Autodesk Inventor part; units mm, degrees
ref_plane "YZ Plane" through (0, 0, 0) normal (1, 0, 0) x (0, 1, 0)
ref_plane "XZ Plane" through (0, 0, 0) normal (0, 1, 0) x (-1, 0, 0)
ref_plane "XY Plane" through (0, 0, 0) normal (0, 0, 1) x (1, 0, 0)
sketch "Sketch1" plane through (0, 0, 0) normal (0, 1, 0) x (-1, 0, 0)
  line L0 (17.0278, 0) -> (-10.5342, 0)
  line L1 (-10.5342, 0) -> (-10.5342, -20.5)
  line L2 (-10.5342, -20.5) -> (17.0278, -20.5)
  line L3 (17.0278, -20.5) -> (17.0278, 0)
  line L4 (4.9658, -15.846) -> (-7.0342, -15.846)
  line L5 (-7.0342, -15.846) -> (-7.0342, -10.846)
  line L6 (-7.0342, -10.846) -> (4.9658, -10.846)
  line L7 (4.9658, -10.846) -> (4.9658, -15.846)
  circle A0 centre (-6.0342, -14.846) radius 1
  circle A1 centre (3.9658, -14.846) radius 1
  circle A2 centre (3.9658, -11.846) radius 1
  circle A3 centre (-6.0342, -11.846) radius 1
  circle A4 centre (-8.5342, -18.5) radius 2
  line L8 (17.0278, -20.5) -> (-8.5342, -20.5)
  line L9 (-8.5342, -20.5) -> (-8.5342, -6.2)
  line L10 (-8.5342, -6.2) -> (17.0278, -6.2)
  line L11 (17.0278, -6.2) -> (17.0278, -20.5)
  line L12 (-10.5342, -20.5) -> (7.4658, -20.5)
  line L13 (7.4658, -20.5) -> (7.4658, -17.5)
  line L14 (7.4658, -17.5) -> (-10.5342, -17.5)
  line L15 (-10.5342, -17.5) -> (-10.5342, -20.5)
  line L16 (7.4658, -17.5) -> (17.0278, -17.5)
  line L17 (17.0278, -17.5) -> (17.0278, -8)
  line L18 (17.0278, -8) -> (7.4658, -8)
  line L19 (7.4658, -8) -> (7.4658, -17.5)
  circle A5 centre (17.0278, -12.75) radius 6.5
  line L20 (17.0278, -17.5) -> (21.4649, -17.5)
  line L21 (21.4649, -17.5) -> (21.4649, -8)
  line L22 (21.4649, -8) -> (17.0278, -8)
  line L23 (17.0278, -8) -> (17.0278, -17.5)
  circle A6 centre (5.6658, -8) radius 1.8
  line L24 (18.4658, -17.5) -> (13.4658, -17.5)
  line L25 (13.4658, -17.5) -> (13.4658, -13.6692)
  line L26 (13.4658, -13.6692) -> (18.4658, -13.6692)
  line L27 (18.4658, -13.6692) -> (18.4658, -17.5)
  circle A7 centre (19.4658, -16.5) radius 1
  circle A8 centre (17.4658, -14.6692) radius 1
  circle A9 centre (14.4658, -14.6692) radius 1
  circle A10 centre (12.4658, -16.5) radius 1
  line L28 (-8.5342, -17.5) -> (-10.5342, -17.5)
  line L29 (-10.5342, -17.5) -> (-10.5342, -6.2)
  line L30 (-10.5342, -6.2) -> (-8.5342, -6.2)
  line L31 (-8.5342, -6.2) -> (-8.5342, -17.5)
  point P0 (0, 0)
  point P1 (4.9658, -11.846)
  point P2 (4.9658, -14.846)
  point P3 (3.9658, -15.846)
  point P4 (-6.0342, -15.846)
  point P5 (-7.0342, -14.846)
  point P6 (-7.0342, -11.846)
  point P7 (-6.0342, -10.846)
  point P8 (3.9658, -10.846)
  point P9 (-8.5342, -16.5)
  point P10 (-8.5342, -20.5)
  point P11 (12.4658, -17.5)
  point P12 (13.4658, -16.5)
  point P13 (13.4658, -14.6692)
  point P14 (14.4658, -13.6692)
  point P15 (17.4658, -13.6692)
  point P16 (18.4658, -14.6692)
  point P17 (18.4658, -16.5)
  point P18 (19.4658, -17.5)
  point P19 (5.6658, -6.2)
  point P20 (-10.5342, -18.5)
  dimension "d26" = 13
  dimension "d1" = 20.5
  dimension "d2" = 0
  dimension "d3" = 12
  dimension "d4" = 5
  dimension "d5" = 4.654
  dimension "d6" = 3.5
  dimension "d7" = 2
  dimension "d8" = 2
  dimension "d9" = 2
  dimension "d10" = 2
  dimension "d11" = 1
  dimension "d12" = 1
  dimension "d13" = 1
  dimension "d14" = 1
  dimension "d15" = 1
  dimension "d16" = 1
  dimension "d17" = 1
  dimension "d18" = 1
  dimension "d19" = 4
  dimension "d20" = 2
  dimension "d21" = 14.3
  dimension "d22" = 18
  dimension "d23" = 3
  dimension "d24" = 9.5
  dimension "d25" = 9.562
  dimension "d27" = 1.8
  dimension "d28" = 5
  dimension "d29" = 8.5
  dimension "d30" = 2
  dimension "d31" = 2
  dimension "d32" = 2
  dimension "d33" = 2
  dimension "d34" = 1
  dimension "d35" = 1
  dimension "d36" = 1
  dimension "d37" = 1
  dimension "d38" = 1
  dimension "d39" = 1
  dimension "d40" = 1
  dimension "d41" = 1
extrude "Extrusion1" add sketch "Sketch1" along normal blind 3 contours L30 L9 A4 L14 L1 | A6 L19 L14 A4 L9 L10 | A6 | L14 A4 L1 | L22 L21 L20 A7 L27 L26 L3 | L3 L26 L25 A10 A5 L18 | A5 L21 | A5 A10 L16 L19 L18 | A4 L14 L9 | A4 L9 L14 | A4 L14 L9 | A10 A5 | A5 A10 | L13 L2 A4 L14 | L9 L14 A4 | A9 L25 L26 | L26 L27 A8 | A7 | L4 A1 L7 | L4 L5 A0 | A2 L6 L7 | L5 L6 A3
mirror "Mirror1" about plane through (0, 0, 0) normal (0, 0, 1) of "Extrusion1"
sketch "Sketch2" plane through (0, 0, 0) normal (0, -1, 0) x (1, 0, 0)
  circle A0 centre (14.5342, -24.5) radius 1
  line L0 (8.5342, -20.5) -> (-7.4658, -20.5)
  line L1 (10.5342, -6.2) -> (10.5342, -18.5)
  line L2 (10.5342, -6.2) -> (16.5342, -6.2)
  line L3 (16.5342, -6.2) -> (16.5342, -28.6617)
  line L4 (16.5342, -28.6617) -> (10.5342, -28.6617)
  line L5 (10.5342, -28.6617) -> (10.5342, -6.2)
  circle A1 centre (14.5342, -24.5) radius 3
  line L6 (8.5342, -20.5) -> (11.5342, -20.5)
  line L7 (11.5342, -20.5) -> (11.5342, -24.5)
  circle A2 centre (9.5342, -22.5) radius 2
  line L8 (16.5342, -6.2) -> (10.5342, -6.2)
  line L9 (10.5342, -6.2) -> (10.5342, 0)
  line L10 (10.5342, 0) -> (16.5342, 0)
  line L11 (16.5342, 0) -> (16.5342, -6.2)
  line L12 (8.5342, -20.5) -> (-7.4658, -20.5)
  line L13 (8.5342, -20.5) -> (10.5342, -18.7057)
  point P0 (0, 0)
  point P1 (9.5342, -20.5)
  point P2 (10.5342, -20.7679)
  point P3 (10.5342, -20.5)
  point P4 (16.5342, -22.2639)
  point P5 (11.5342, -22.5)
  dimension "d48" = 6
  dimension "d44" = 2
  dimension "d46" = 4
  dimension "d47" = 6
  dimension "d49" = 4
  dimension "d50" = 2
  dimension "d51" = 6.2
  dimension "d64" = 24.5
extrude "Extrusion2" add sketch "Sketch2" against normal blind 3 contours L2 L3 A1 L7 L6 L5 L1 | L9 L10 L11 L2 | L5 L6 L13 | A1 L3 | L3 A1 | L6 L7 A2 L5 | L5 A2 L6
mirror "Mirror2" about plane through (10.5342, 0, 0) normal (0, 0, 1) of "Extrusion2"
sketch "Sketch3" plane through (0, 0, 0) normal (0, -1, 0) x (1, 0, 0)
  line L0 (13.5342, 15.5) -> (16.5342, 15.5)
  line L1 (16.5342, 15.5) -> (16.5342, -15.5)
  line L2 (16.5342, -15.5) -> (13.5342, -15.5)
  line L3 (13.5342, -15.5) -> (13.5342, 15.5)
  line L4 (16.5342, -22.2639) -> (16.5342, 22.2639)
  point P0 (0, 0)
  dimension "d54" = 31
  dimension "d55" = 0
  dimension "d56" = 15.5
  dimension "d57" = 3
extrude "Extrusion3" cut sketch "Sketch3" against normal blind 3
sketch "Sketch5" plane through (0, 0, 0) normal (0, -1, 0) x (1, 0, 0)
  line L0 (10.5342, 6.5) -> (-20.8216, 6.5)
  line L1 (-20.8216, 6.5) -> (-20.8216, -6.5)
  line L2 (-20.8216, -6.5) -> (10.5342, -6.5)
  line L3 (10.5342, -6.5) -> (10.5342, 6.5)
  point P0 (0, 0)
  dimension "d60" = 13
  dimension "d61" = 6.5
extrude "Extrusion4" cut sketch "Sketch5" against normal blind 3
sketch "Sketch6" plane through (0, 3, 0) normal (0, 1, 0) x (1, 0, 0)
  line L0 (9.5342, 20.5) -> (-7.4658, 20.5)
  line L1 (-6.6608, 6.5) -> (10.5342, 6.5)
  line L2 (7.0342, 20.5) -> (9.0342, 20.5)
  line L3 (9.0342, 20.5) -> (9.0342, 6.5)
  line L4 (9.0342, 6.5) -> (7.0342, 6.5)
  line L5 (7.0342, 6.5) -> (7.0342, 20.5)
  line L6 (10.5342, 6.5) -> (10.5342, -6.5)
  line L7 (7.0342, 14.846) -> (7.0342, 11.846)
  point P0 (0, 0)
  dimension "d65" = 1.5
  dimension "d66" = 0
extrude "Extrusion5" add sketch "Sketch6" along normal blind 3
mirror "Mirror3" about plane through (0, 0, 0) normal (0, 0, 1) of "Extrusion5"
properties part number "Base_modded"
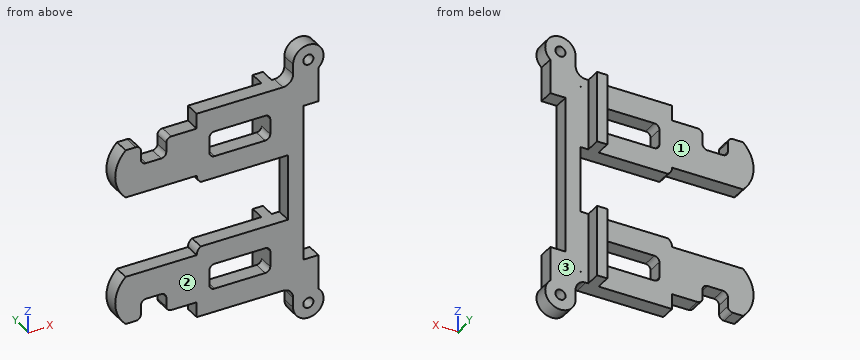
Geometry check sheet. Reference: the model listing, model coordinates, mm. Face numbers are marked on the shaded views. A direction names the side the tool comes from. Give positions to 0.01 mm unless a question says otherwise; leave off trailing zeros. Loops run counter-clockwise (first coordinate to the right, second up) from the corner with the lowest first, then second, coordinate; pieces in that order, holes last.
(1) Set-up check for the marked faces 1, 2 and 3: record each of +Z, -Z, +X, -X, +Y, -Y from which the full face is reachable in a straight line by a thin tool's end or side.
From the geometry:
face 1: +Z, -Z, -X, +Y
face 2: +Z, -Z, +X, -X, -Y
face 3: +Z, -Z, +X, +Y
(2) Section check B-B on z = 3. Record the cut outline in (x, y), then the cut area to 3 significant figures.
From the geometry:
outline: (10.53, 0) - (13.53, 0) - (13.53, 3) - (10.53, 3) - close
area: 9.00 mm2
(3) Depth check by flat-ended pin: pin 1 Ø2.5 at (x, y) = (-16.5, 2) entering from +Z; pin 2 Ø0.9 at (x, y) = (-10.5, 1) entering from -Z; pin 3 Ø1 at (y, z) = (4, -7) entering from +X. Enter the tip coordinate at first touch or a pass-through.
From the geometry:
pin 1: stops at z = 13.71
pin 2: stops at z = -17.5
pin 3: stops at x = 9.03
(4) Section check A-A on x = -6. Record the cut outline in (y, z).
From the geometry:
outline: (0, -20.5) - (3, -20.5) - (3, -6.5) - (0, -6.5) - close; (0, 6.5) - (3, 6.5) - (3, 20.5) - (0, 20.5) - close
(5) Section check C-C on y = 1.75. Count the separate pieces of the cut face and the enclosed holes in it, then the cut area to 3 significant figures.
From the geometry:
separate pieces: 1
enclosed holes: 6
area: 860 mm2
(6) Thickness scan on L1, parallel to Z at x = 14.5, y = 2.65; L2, parallel to Z at x = -0.5, y = 2.8; L3, parallel to X at y = 1.1, z = 24.5. Record the ranges inside material, lowest first.
From the geometry:
L1: z = -27.5 to -25.5, -23.5 to -15.5, 15.5 to 23.5, 25.5 to 27.5
L2: z = -20.5 to -15.85, -10.85 to -6.5, 6.5 to 10.85, 15.85 to 20.5
L3: x = 11.53 to 13.53, 15.53 to 17.53
